Could you check a few things on this model? Use its own coordinates, in mm. Face numbers are marked on the shaded views. A direction names the side the tool comes from. Round coordinates to 2 decimals unless told otherwise and drop trailing zeros. Loops run counter-clockwise (first coordinate to the right, second up) from the corner with the lowest first, then second, coordinate; pieces in that order, holes last. Notation, with made-up numbers: (64.5, -24) - (109.5, -24) arc R8 ccw to (109.5, -19) - close; hole circle Ø10 at (35, -35.75). An arc over 180 degrees is marked (long way). Answer as CSV lines item,"result". Start each with the question number.
1) Suppose I cut it at B-B, the plane z = -11. Write out the boundary of the cut face in (x, y).
2) Suppose I cut it at C-C, the plane y = 12.5. Write out the boundary of the cut face in (x, z).
3) Suppose I cut it at D-D, the plane x = 22. Write out the boundary of the cut face in (y, z).
4) We'd pull the mould along X, two halves only. Please class the marked faces 3, 4, 5 and 6: pulls with the +X half, pulls with the -X half, needs draft (parallel to the pull), parting line crosses it, or undercut.
5) I'm going to push flat-ended pins straight in: pin 1 Ø8 at (x, y) = (16, 3.5) entering from +Z; pin 2 Ø3 at (x, z) = (27.5, -31.5) entering from +Y. Where does each tip first touch, or does it pass through?
6) Which directions (+Z, -Z, +X, -X, +Y, -Y) give clear straight access to the entire face, cutting with the end or side of a thin tool? Please do the marked faces 1 and 2.
7) Suppose I cut it at A-A, the plane y = 7.5. Write out the boundary of the cut face in (x, z).
8) Please list where these lines run through material, in increasing order: line 1 along X through (y, z) = (3, -20.5); line 2 along Z through (x, y) = (3.5, 3.5); line 3 along Z through (x, y) = (32.5, 7).
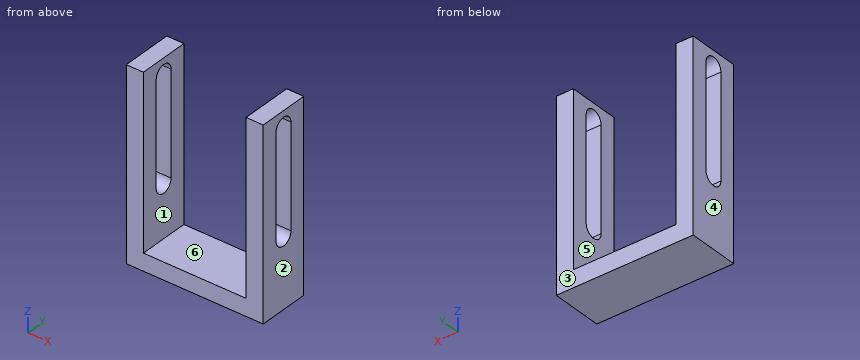
```python
from build123d import *

# Parameters (mm, degrees)
BOSS_EXTRUDE1_DEPTH = 15
CUT_EXTRUDE1_DEPTH  = 41


with BuildPart() as part:
    # Sketch1 → Boss-Extrude1 (new body)
    with BuildSketch(Plane(origin=(0, 0, 0), x_dir=(1, 0, 0), z_dir=(0, 1, 0))):
        Polygon((0, 0), (-5, 0), (-5, 55), (23.965517241, 55), (35, 55), (35, 0), (30, 0), (30, 50), (0, 50), align=None)
    extrude(amount=BOSS_EXTRUDE1_DEPTH)

    # Sketch2 → Cut-Extrude1 (cut, through all)
    with BuildSketch(Plane(origin=(35, 0, 0), x_dir=(0, 0, -1), z_dir=(1, 0, 0))):
        with BuildLine():
            Line((4.564965869, 10.25), (34.659838249, 10.25))
            ThreePointArc((34.659838249, 10.25), (37.409838249, 7.5), (34.659838249, 4.75))
            Line((34.659838249, 4.75), (4.564965869, 4.75))
            ThreePointArc((4.564965869, 4.75), (1.814965869, 7.5), (4.564965869, 10.25))
        make_face()
    extrude(amount=-CUT_EXTRUDE1_DEPTH, mode=Mode.SUBTRACT)


solid = part.part
```
Filled sheet:
1,outline,"(-5, 0) - (0, 0) - (0, 4.75) - (-5, 4.75) - close; (-5, 10.25) - (0, 10.25) - (0, 15) - (-5, 15) - close; (30, 0) - (35, 0) - (35, 4.75) - (30, 4.75) - close; (30, 10.25) - (35, 10.25) - (35, 15) - (30, 15) - close"
2,outline,"(-5, -55) - (35, -55) - (35, 0) - (30, 0) - (30, -50) - (0, -50) - (0, 0) - (-5, 0) - close"
3,outline,"(0, -55) - (15, -55) - (15, -50) - (0, -50) - close"
4,face 3,"needs draft"
4,face 4,"pulls with the -X half"
4,face 5,"undercut"
4,face 6,"undercut"
5,pin 1,"z = -50"
5,pin 2,"through"
6,face 1,"+Z, +Y, -Y"
6,face 2,"+Z, -Z, +X, +Y, -Y"
7,outline,"(-5, -55) - (35, -55) - (35, -37.41) - (30, -37.41) - (30, -50) - (0, -50) - (0, -37.41) - (-5, -37.41) - close; (-5, -1.81) - (0, -1.81) - (0, 0) - (-5, 0) - close; (30, -1.81) - (35, -1.81) - (35, 0) - (30, 0) - close"
8,line 1,"-5 to 0, 30 to 35"
8,line 2,"-55 to -50"
8,line 3,"-55 to -37.36, -1.86 to 0"
